The listing builds one solid part. Answer for the finished solid, in the listing's coordinates (mm). A direction names the side the tool comes from. Give positions to 0.01 mm unless a question says otherwise; leave off trailing zeros. Write each loop counter-clockwise with the first axis right and the second up, starting at its lowest first coordinate (ties: lowest second). Pieces come first, ordered by that corner, then holes. Notation, with made-up numbers: (-18.75, 89.5) - (9.25, 89.5) arc R29 ccw to (9.25, 109.5) - close; hole circle Ø7 at (57, 87.5). An arc over 180 degrees is marked (long way). One line per item, written item: value. Start each with the question number.
from build123d import *

# Parameters (mm, degrees)
SALIENTE_EXTRUIR1_DEPTH             = 7.21
SALIENTE_EXTRUIR2_DEPTH             = 7.21
SALIENTE_EXTRUIR2_DEPTH_BACK        = 7.21
CORTAR_EXTRUIR2_DEPTH               = 28.232395202
CORTAR_EXTRUIR2_DEPTH_BACK          = 28.232395202
SALIENTE_EXTRUIR3_REACH             = 29.232
SALIENTE_EXTRUIR3_DIRECTION_2_REACH = 29.232


with BuildPart() as part:
    # Croquis1 → Saliente-Extruir1 (new, symmetric)
    with BuildSketch(Plane.XY):
        with BuildLine():
            add(Edge.make_bspline(
                [(-18.945192114, 7.540918896), (-10.215008384, -3.697644103), (-2.846604825, -5.059081104)],
                knots=[0.497667241, 0.497667241, 0.497667241, 0.49955428, 0.49955428, 0.49955428], degree=2, weights=[1, 1, 1]))
            add(Edge.make_bspline(
                [(-2.846604825, -5.059081104), (-0.742366882, -3.9352066), (0.355125, -2.723253227)],
                knots=[0.498812075, 0.498812075, 0.498812075, 0.499412845, 0.499412845, 0.499412845], degree=2, weights=[1, 1, 1]))
            Line((0.355125, -2.723253227), (0.355125, -2.284841781))
            Line((0.355125, -2.284841781), (-1.394875, -2.223730435))
            add(Edge.make_bspline(
                [(-1.394875, -2.223730435), (-0.90753067, -0.123730435), (-1.394875, 1.976269565)],
                knots=[0, 0, 0, 1, 1, 1], degree=2, weights=[1, 3.231801219, 1]))
            Line((-1.394875, 1.976269565), (0.355125, 2.284841781))
            Line((0.355125, 2.284841781), (0.355125, 3.001549529))
            add(Edge.make_bspline(
                [(0.355125, 3.001549529), (-1.44872627, 6.058427314), (-6.994875026, 10.477389992)],
                knots=[0.500820705, 0.500820705, 0.500820705, 0.502013312, 0.502013312, 0.502013312], degree=2, weights=[1, 1, 1]))
            Line((-6.994875026, 10.477389992), (-8.981845695, 12.608155172))
            Line((-8.981845695, 12.608155172), (-23.035921146, 11.871612288))
            Line((-23.035921146, 11.871612288), (-23.035921146, 11.54013782))
            ThreePointArc((-23.035921146, 11.54013782), (-20.949684518, 9.582335705), (-18.945192114, 7.540918896))
        make_face()
    extrude(amount=SALIENTE_EXTRUIR1_DEPTH, both=True)

    # Croquis4 → Saliente-Extruir2 (add, two sides: drawn at the far end of the back side and taken through both)
    with BuildSketch(Plane.XY.offset(-SALIENTE_EXTRUIR2_DEPTH_BACK)):
        Polygon((-1.394875, 1.976269565), (0.355125, 2.284841781), (0.355125, 1.976269565), align=None)
    extrude(amount=SALIENTE_EXTRUIR2_DEPTH + SALIENTE_EXTRUIR2_DEPTH_BACK)

    # Croquis6 → Cortar-Extruir2 (cut, two sides: drawn at the far end of the back side and taken through both)
    with BuildSketch(Plane(origin=(0, 0, 0), x_dir=(0, 0, -1), z_dir=(1, 0, 0)).offset(-CORTAR_EXTRUIR2_DEPTH_BACK)):
        Polygon((7.21, 12.608155172), (7.21, -5.059081104), (5.21, -5.059081104), align=None)
        Polygon((-7.21, 12.608155172), (-7.21, -5.059081104), (-5.21, -5.059081104), align=None)
    extrude(amount=CORTAR_EXTRUIR2_DEPTH + CORTAR_EXTRUIR2_DEPTH_BACK, mode=Mode.SUBTRACT)

    # Saliente-Extruir3: up to this plane
    saliente_extruir3_end = Plane(origin=(-23.035921146, 12.608155172, 7.21), z_dir=(0, 0.1124854344122626, -0.9936533736897816))
    # Croquis8 → Saliente-Extruir3 (add, up to the surface)
    with BuildSketch(Plane.XY, mode=Mode.PRIVATE) as saliente_extruir3_sk1:
        with BuildLine():
            Line((-6.40174466, 10), (0.355125, 10))
            Line((0.355125, 10), (0.355125, 3.001549529))
            add(Edge.make_bspline(
                [(-6.40174466, 10), (-1.350464373, 5.891908813), (0.355125, 3.001549529)],
                knots=[0.50088567, 0.50088567, 0.50088567, 0.502013312, 0.502013312, 0.502013312], degree=2, weights=[1, 1, 1]))
        make_face()
    saliente_extruir3_tool1 = split(extrude(saliente_extruir3_sk1.sketch, amount=SALIENTE_EXTRUIR3_REACH, mode=Mode.PRIVATE), bisect_by=saliente_extruir3_end, keep=Keep.BOTH, mode=Mode.PRIVATE)
    add(saliente_extruir3_tool1.solids().sort_by_distance((-1.802267, 7.821617, 0))[0])

    # Saliente-Extruir3 direction 2: up to this plane
    saliente_extruir3_direction_2_end = Plane(origin=(-23.035921146, 12.608155172, -7.21), z_dir=(0, 0.1124854344122626, 0.9936533736897816))
    # Croquis8 → Saliente-Extruir3 direction 2 (add, up to the surface)
    with BuildSketch(Plane.XY, mode=Mode.PRIVATE) as saliente_extruir3_direction_2_sk1:
        with BuildLine():
            Line((-6.40174466, 10), (0.355125, 10))
            Line((0.355125, 10), (0.355125, 3.001549529))
            add(Edge.make_bspline(
                [(-6.40174466, 10), (-1.350464373, 5.891908813), (0.355125, 3.001549529)],
                knots=[0.50088567, 0.50088567, 0.50088567, 0.502013312, 0.502013312, 0.502013312], degree=2, weights=[1, 1, 1]))
        make_face()
    saliente_extruir3_direction_2_tool1 = split(extrude(saliente_extruir3_direction_2_sk1.sketch, amount=-SALIENTE_EXTRUIR3_DIRECTION_2_REACH, mode=Mode.PRIVATE), bisect_by=saliente_extruir3_direction_2_end, keep=Keep.BOTH, mode=Mode.PRIVATE)
    add(saliente_extruir3_direction_2_tool1.solids().sort_by_distance((-1.802267, 7.821617, 0))[0])


solid = part.part
Item 1: Find section A-A on y = 9. Determine the outline of the cut face in (x, z), plus the area to 3 significant figures.
Item 2: The mould has two halves that part along Y. Classify faces 3 (the flat face through (0.355, 6, 0)), 4 (the flat face through (-15.911, 12.245, 0.101)), 5 (the flat face through (-1, 1.976, 0)), 6 (the flat face through (-8.905, 5.861, 6.446)): +Y half, -Y half, draft (parallel to the pull), parting line (faces both ways), or undercut.
Item 3: Each of these flat-tipped pins is pushed along its axis until it touches: pin 1 Ø3 at (x, z) = (-19.5, 5.5) entering from -Y; pin 2 Ø1 at (x, z) = (-20, -4.5) entering from +Y; pin 3 Ø2 at (x, z) = (-13, -2) entering from -Y. Where does it stop, or does it pass through?
Item 4: Straight lines are drawn through the part: line 1 along Z through (x, y) = (-18.75, 7.5); line 2 along X through (y, z) = (9, 6.25); line 3 along Z through (x, y) = (-6.5, 3.25). For each, find the intervals that lie inside material, in ascending order.
Item 5: For faces 1 (the flat face through (-8.905, 5.614, -6.418)), 2 (the flat face through (-3, 10, 0)), determine the directions among +Z, -Z, +X, -X, +Y, -Y from which every point of the face is accessible in a straight line to the end or side of a thin tool.
Values:
1. outline: (-20.36, -6.8) - (0.36, -6.8) - (0.36, 6.8) - (-20.36, 6.8) - close
1. area: 282 mm^2
2. face 3: draft
2. face 4: +Y half
2. face 5: undercut
2. face 6: -Y half
3. pin 1: y = 6.35
3. pin 2: y = 12.06
3. pin 3: y = -0.03
4. line 1: -6.63 to 6.63
4. line 2: -20.36 to 0.36
4. line 3: -6.15 to 6.15
5. face 1: -Z, +X, -X, -Y
5. face 2: +Z, -Z, +X, +Y
